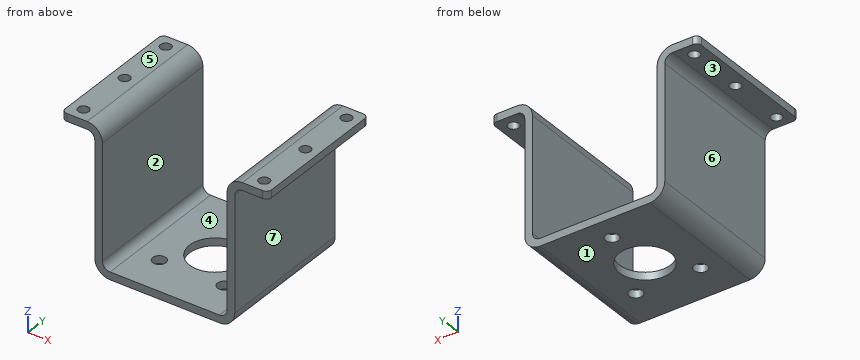
Autodesk Inventor part; units mm, degrees
ref_plane "YZ Plane" through (0, 0, 0) normal (1, 0, 0) x (0, 1, 0)
ref_plane "XZ Plane" through (0, 0, 0) normal (0, 1, 0) x (-1, 0, 0)
ref_plane "XY Plane" through (0, 0, 0) normal (0, 0, 1) x (1, 0, 0)
sketch "スケッチ1" plane through (0, 0, 0) normal (0, 0, 1) x (1, 0, 0)
  line L0 (27.5, -27.5) -> (-27.5, -27.5)
  line L1 (-27.5, -27.5) -> (-27.5, 27.5)
  line L2 (-27.5, 27.5) -> (27.5, 27.5)
  line L3 (27.5, 27.5) -> (27.5, -27.5)
  line L4 (27.5, -27.5) -> (-27.5, 27.5) construction
  line L5 (-27.5, -27.5) -> (27.5, 27.5) construction
  point P0 (0, 0)
  dimension "d0" = 55
  dimension "d1" = 55
extrude "プレート1" add sketch "スケッチ1" along normal blind 3
sketch "スケッチ2" plane through (0, 0, 3) normal (0, 0, 1) x (1, 0, 0)
  line L0 (-27.5, -27.5) -> (-27.5, 27.5)
  line L1 (27.5, -27.5) -> (-27.5, -27.5)
  line L2 (27.5, 27.5) -> (27.5, -27.5)
  line L3 (-27.5, 27.5) -> (27.5, 27.5)
  circle A0 centre (0, 0) radius 18
  point P0 (0, 18)
  point P1 (-18, 0)
  point P2 (0, -18)
  point P3 (18, 0)
  point P4 (-12.728, -12.7278)
  point P5 (12.728, -12.7278)
  dimension "d3" = 36
  dimension "d54" = 25.456
hole "穴1" at (0, 18, 3) at (12.728, -12.7278, 3) at (-12.728, -12.7278, 3) direction (0, 0, -1) diameter 5.2 end through all
sketch "スケッチ3" plane through (0, 0, 3) normal (0, 0, 1) x (1, 0, 0)
  circle A0 centre (0, 0) radius 10
  dimension "d15" = 20
extrude "押し出し1" cut sketch "スケッチ3" against normal blind 10
sketch "スケッチ4" plane through (-24.5, -27.5, 0) normal (-1, 0, 0) x (0, -1, 0)
  line L0 (-55, 0) -> (0, 0)
  line L1 (0, 0) -> (0, 57)
  line L2 (0, 57) -> (-55, 57)
  line L3 (-55, 57) -> (-55, 0)
edge flange "フランジ1" height 57 angle 90 thickness 3 bend radius 3 thickness toward (-1, 0, 0) relief tear relief width 3 relief depth 1.5 corner gap 3 corner form 0 edges at (-27.5, 0, 3) (27.5, 0, 3) wall of the first edge with corners at (-24.5, 27.5, 0) (-24.5, -27.5, 0) (-24.5, -27.5, 57) (-24.5, 27.5, 57)
bend "曲げ1"
corner "コーナー1"
sketch "スケッチ5" plane through (24.5, -27.5, 54) normal (0, 0, 1) x (1, 0, 0)
  line L0 (0, 55) -> (0, 0)
  line L1 (0, 0) -> (16, 0)
  line L2 (16, 0) -> (16, 55)
  line L3 (16, 55) -> (0, 55)
edge flange "フランジ2" height 16 angle 90 thickness 3 bend radius 3 thickness toward (0, 0, 1) relief tear relief width 3 relief depth 1.5 corner gap 3 corner form 0 edges at (27.5, 0, 57) (-27.5, 0, 57) wall of the first edge with corners at (24.5, 27.5, 54) (24.5, -27.5, 54) (40.5, -27.5, 54) (40.5, 27.5, 54)
bend "曲げ2"
corner "コーナー2"
fillet "フィレット1" radius 2 4 edges at (40.5, 27.5, 55.5) (40.5, -27.5, 55.5) (-40.5, -27.5, 55.5) (-40.5, 27.5, 55.5)
sketch "スケッチ8" plane through (-30.5, -27.5, 57) normal (0, 0, 1) x (1, 0, 0)
  arc A0 (-8, 55) -> (-10, 53) centre (-8, 53) ccw
  line L0 (-10, 2) -> (-10, 53)
  arc A1 (-10, 2) -> (-8, 0) centre (-8, 2) ccw
  line L1 (0, 0) -> (-8, 0)
  line L2 (0, 0) -> (0, 55)
  line L3 (-8, 55) -> (0, 55)
  arc A2 (69, 0) -> (71, 2) centre (69, 2) ccw
  line L4 (71, 53) -> (71, 2)
  arc A3 (71, 53) -> (69, 55) centre (69, 53) ccw
  line L5 (61, 55) -> (69, 55)
  line L6 (61, 55) -> (61, 0)
  line L7 (69, 0) -> (61, 0)
  line L8 (-5, 50) -> (66, 50)
  line L9 (66, 50) -> (66, 5)
  line L10 (66, 5) -> (-5, 5)
  line L11 (-5, 5) -> (-5, 50)
  point P0 (30.5, 27.5)
  point P1 (-5, 27.5)
  point P2 (66, 27.5)
  dimension "d55" = 5
  dimension "d56" = 5
  dimension "d57" = 5
  dimension "d58" = 5
hole "穴3" at (-35.5, 0, 57) at (35.5, 0, 57) at (-35.5, -22.5, 57) at (-35.5, 22.5, 57) at (35.5, -22.5, 57) at (35.5, 22.5, 57) direction (0, 0, -1) diameter 4.2 end through all
equation "\"d13\" = Thickness"
equation "\"d64\" = Thickness"
equation "\"d2\" = Thickness"
equation "\"d18\" = BendReliefWidth"
equation "\"d19\" = BendReliefDepth"
equation "\"d20\" = MinimumRemnant"
equation "\"d21\" = TransitionRadius"
equation "\"d24\" = BendRadius"
equation "\"d25\" = CornerReliefSize"
equation "\"d26\" = GapSize"
equation "\"d27\" = JacobiRadiusSize"
equation "\"d28\" = BendReliefWidth"
equation "\"d29\" = BendReliefDepth"
equation "\"d30\" = MinimumRemnant"
equation "\"d31\" = TransitionRadius"
equation "\"d34\" = BendRadius"
equation "\"d35\" = CornerReliefSize"
equation "\"d36\" = GapSize"
equation "\"d37\" = JacobiRadiusSize"
equation "\"BendRadius\" = Thickness"
equation "\"BendReliefWidth\" = Thickness"
equation "\"BendReliefDepth\" = 0.5 * Thickness"
equation "\"CornerReliefSize\" = 4 * Thickness"
equation "\"MinimumRemnant\" = 2 * Thickness"
equation "\"TransitionRadius\" = BendRadius"
equation "\"JacobiRadiusSize\" = BendRadius"
equation "\"GapSize\" = Thickness"
properties part number "CCM_Motor_Mount_A"
Model file for the job. Use its own axes, mm. Face numbers are marked on the shaded views. A direction names the side the tool comes from. Give positions to 0.01 mm unless a question says otherwise; leave off trailing zeros. Write each loop counter-clockwise with the first axis right and the second up, starting at its lowest first coordinate (ties: lowest second). Pieces come first, ordered by that corner, then holes. Notation, with made-up numbers: (-22.5, -37.5) - (4.5, -37.5) arc R12 cw to (4.5, -33.5) - close; hole circle Ø3 at (81, 60.25). An arc over 180 degrees is marked (long way). One line per question, with ' | ' between items. Start each with the question number.
(1) 3-axis set-ups, long thin cutter, end or side, ignore diameter. For the marked faces 1, 2 and 3: which of +Z, -Z, +X, -X, +Y, -Y reach the whole face in a straight line?
(2) Wall check: line 1 along Y through (x, z) = (-35.5, 55.45); line 2 along X through (y, z) = (24, 7.5); line 3 along Z through (x, y) = (-13, -2). Give the ranges that are in metal, low to high. Write a range as from..to.
(3) Slice it at A-A on x = 0. Write the cut outline in (y, z).
(4) Slice it at C-C on x = 35.5. Write the cut outline in (y, z), plus the area to 3 significant figures.
(5) Slice it at B-B on y = 22.5. Write the cut outline in (x, z).
(6) Two-plate mould, pull along X, no slides. Class the marked faces 4, 5, 6 and 7: +X half, -X half, draft (parallel to the pull), parting line (faces both ways), or undercut.
(7) Pin check, flat tips, straight feed: P1, Ø5, axis at x = 28, y = 18, coming from the -Z side; P2, Ø13.5, axis at y = -10, z = 25.5, coming from the +X side; P3, Ø12, axis at x = 24, y = 1, coming from the +Z side; P4, Ø2.5, axis at x = 35.5, y = 0, coming from the -Z side. Stop position of each tip, or through.
(8) Slice it at D-D on z = 34. Write the cut outline in (x, y).
Results below:
1) face 1: -Z, +X, -X, +Y, -Y | face 2: +Z, +Y, -Y | face 3: -Z, -X, +Y, -Y
2) line 1: -27.5..-24.6, -20.4..-2.1, 2.1..20.4, 24.6..27.5 | line 2: -27.5..-24.5, 24.5..27.5 | line 3: 0..3
3) outline: (-27.5, 0) - (-10, 0) - (-10, 3) - (-27.5, 3) - close; (10, 0) - (15.4, 0) - (15.4, 3) - (10, 3) - close; (20.6, 0) - (27.5, 0) - (27.5, 3) - (20.6, 3) - close
4) outline: (-27.5, 54) - (-24.6, 54) - (-24.6, 57) - (-27.5, 57) - close; (-20.4, 54) - (-2.1, 54) - (-2.1, 57) - (-20.4, 57) - close; (2.1, 54) - (20.4, 54) - (20.4, 57) - (2.1, 57) - close; (24.6, 54) - (27.5, 54) - (27.5, 57) - (24.6, 57) - close | area: 127 mm^2
5) outline: (-40.5, 54) - (-37.6, 54) - (-37.6, 57) - (-40.5, 57) - close; (-33.4, 54) - (-30.5, 54) arc R3 cw to (-27.5, 51) - (-27.5, 6) arc R6 ccw to (-21.5, 0) - (21.5, 0) arc R6 ccw to (27.5, 6) - (27.5, 51) arc R3 cw to (30.5, 54) - (33.4, 54) - (33.4, 57) - (30.5, 57) arc R6 ccw to (24.5, 51) - (24.5, 6) arc R3 cw to (21.5, 3) - (-21.5, 3) arc R3 cw to (-24.5, 6) - (-24.5, 51) arc R6 ccw to (-30.5, 57) - (-33.4, 57) - close; (37.6, 54) - (40.5, 54) - (40.5, 57) - (37.6, 57) - close
6) face 4: undercut | face 5: draft | face 6: -X half | face 7: +X half
7) P1: z = 1.53 | P2: x = 27.5 | P3: z = 56.98 | P4: through
8) outline: (-27.5, -27.5) - (-24.5, -27.5) - (-24.5, 27.5) - (-27.5, 27.5) - close; (24.5, -27.5) - (27.5, -27.5) - (27.5, 27.5) - (24.5, 27.5) - close
